Geometry check sheet. Reference: the model listing, model coordinates, mm. Face numbers are marked on the shaded views. A direction names the side the tool comes from. Coordinates: 2 decimals unless noted, no trailing zeros. Loops run counter-clockwise (first coordinate to the right, second up) from the corner with the lowest first, then second, coordinate; pieces in that order, holes last.
from build123d import *

# Parameters (mm, degrees)
SKETCH1_W                            = 6
SKETCH1_H                            = 3.5
SKETCH1_R                            = 0.36
SKETCH1_R_2                          = 0.63
CANULALAYOUT_BOSS_EXTRUDE1_DEPTH     = 5.5
SKETCH2_W                            = 16
SKETCH2_H                            = 7.5
SKETCH2_R                            = 0.25
BASE_BOSS_EXTRUDE2_DEPTH             = 2
SKETCH3_R                            = 0.63
SKETCH3_R_2                          = 0.25
HEIGHTDIFFERENCE_BOSS_EXTRUDE3_DEPTH = 0.2


with BuildPart() as part:
    # Sketch1 → CanulaLayout-Boss-Extrude1 (new body)
    with BuildSketch(Plane(origin=(0, 0, 0), x_dir=(1, 0, 0), z_dir=(0, 1, 0))):
        Rectangle(SKETCH1_W, SKETCH1_H)
        with Locations(Location((1.072966062, 0.541981393, 0), (0, 0, 270))):
            Circle(SKETCH1_R, mode=Mode.SUBTRACT)
        with Locations(Location((2.109800031, -0.541981393, 0), (0, 0, 270))):
            Circle(SKETCH1_R, mode=Mode.SUBTRACT)
        with Locations(Location((-1.591383046, 0, 0), (0, 0, 270))):
            Circle(SKETCH1_R_2, mode=Mode.SUBTRACT)
    extrude(amount=CANULALAYOUT_BOSS_EXTRUDE1_DEPTH)

    # Sketch2 → Base-Boss-Extrude2 (add)
    with BuildSketch(Plane.XZ):
        Rectangle(SKETCH2_W, SKETCH2_H)
        with Locations(Location((2.109800031, 0.541981393, 0), (0, 0, 270))):
            Circle(SKETCH2_R, mode=Mode.SUBTRACT)
        with Locations(Location((1.072966062, -0.541981393, 0), (0, 0, 270))):
            Circle(SKETCH2_R, mode=Mode.SUBTRACT)
        with Locations(Location((-1.591383046, 0, 0), (0, 0, 270))):
            Circle(SKETCH2_R, mode=Mode.SUBTRACT)
    extrude(amount=BASE_BOSS_EXTRUDE2_DEPTH)

    # Sketch3 → HeightDifference-Boss-Extrude3 (add)
    with BuildSketch(Plane(origin=(0, 0, 0), x_dir=(1, 0, 0), z_dir=(0, 1, 0))):
        with Locations(Location((-1.591383046, 0, 0), (0, 0, 270))):
            Circle(SKETCH3_R)
        with Locations(Location((-1.591383046, 0, 0), (0, 0, 270))):
            Circle(SKETCH3_R_2, mode=Mode.SUBTRACT)
    extrude(amount=HEIGHTDIFFERENCE_BOSS_EXTRUDE3_DEPTH)


solid = part.part
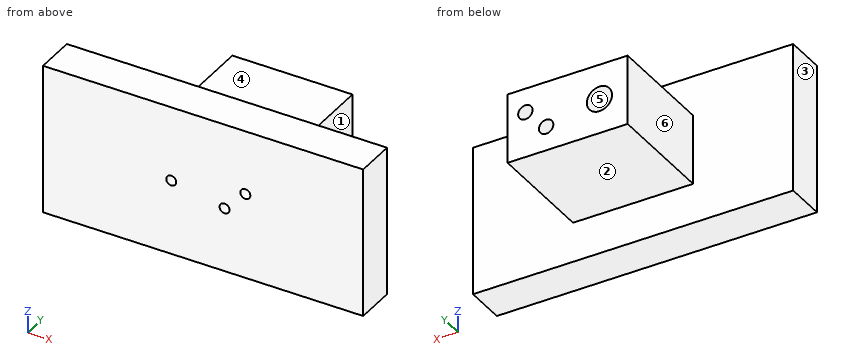
1) Access from +Z, -Z, +X, -X, +Y, -Y to the whole of each face (thin tool, end or side, straight path). Record for the marked faces 1, 2 and 3.
Data:
face 1: +Z, -Z, +X, +Y
face 2: -Z, +X, -X, +Y
face 3: +Z, -Z, -X, +Y, -Y
2) Mould release check, pull along X, two halves, no side actions. Record for the marked faces 4, 5 and 6: +X half, -X half, draft (parallel to the pull), parting line (faces both ways), or undercut.
Data:
face 4: draft
face 5: undercut
face 6: -X half
3) Section check A-A on z = 0. Record the cut outline in (x, y), and give its area (3 significant figures).
Data:
outline: (-8, -2) - (-1.84, -2) - (-1.84, 0.2) - (-2.22, 0.2) - (-2.22, 5.5) - (-3, 5.5) - (-3, 0) - (-8, 0) - close; (-1.34, -2) - (8, -2) - (8, 0) - (3, 0) - (3, 5.5) - (-0.96, 5.5) - (-0.96, 0.2) - (-1.34, 0.2) - close
area: 57.2 mm2
4) Depth check by flat-ended pin: pin 1 (3 mm diameter, centred on x = -1, y = 3, fed in from +Z); pin 2 (1 mm diameter, centred on y = 3.5, z = 0, fed in from -X); pin 3 (1 mm diameter, centred on y = 2.5, z = 0, fed in from +X). Enter the tip coordinate at first touch or a pass-through.
Data:
pin 1: stops at z = 1.75
pin 2: stops at x = -3
pin 3: stops at x = 3
5) Section check D-D on z = 1.25. Record the cut outline in (x, y).
Data:
outline: (-8, -2) - (8, -2) - (8, 0) - (3, 0) - (3, 5.5) - (-3, 5.5) - (-3, 0) - (-8, 0) - close
6) Section check C-C on x = -0.75. Record the cut outline in (y, z), and give its area (4 significant figures).
Data:
outline: (-2, -3.75) - (0, -3.75) - (0, -1.75) - (5.5, -1.75) - (5.5, 1.75) - (0, 1.75) - (0, 3.75) - (-2, 3.75) - close
area: 34.25 mm2
7) Section check B-B on y = 3. Record the cut outline in (x, z), and give its area (3 significant figures).
Data:
outline: (-3, -1.75) - (3, -1.75) - (3, 1.75) - (-3, 1.75) - close; hole circle Ø1.26 at (-1.59, 0); hole circle Ø0.72 at (1.07, -0.54); hole circle Ø0.72 at (2.11, 0.54)
area: 18.9 mm2
8) Material ranges on probe 1 along X at (y, z) = (4.4, 0); probe 2 along Z at (x, y) = (0, 0.5); probe 3 along Y at (x, z) = (1.25, 3), recorded low to high.
Data:
probe 1: x = -3 to -2.22, -0.96 to 3
probe 2: z = -1.75 to 1.75
probe 3: y = -2 to 0
